Could you check a few things on this drawing? It's one solid part, dimensions in mm from its lowest x, y, z. Coordinates: 2 decimals unless noted, no trailing zeros. Order: outer loops, then holes, each group sorted by start corner. A loop starts at its lowest first (then second) coordinate and runs counter-clockwise, first axis right, second up. Notation, with made-up numbers: (71.5, 62.25) -> (127.5, 62.25) arc R20 cw to (127.5, 93.25) -> close; hole circle Ø9 at (77, -25). An arc over 180 degrees is marked (long way). Answer as CSV lines item,"result".
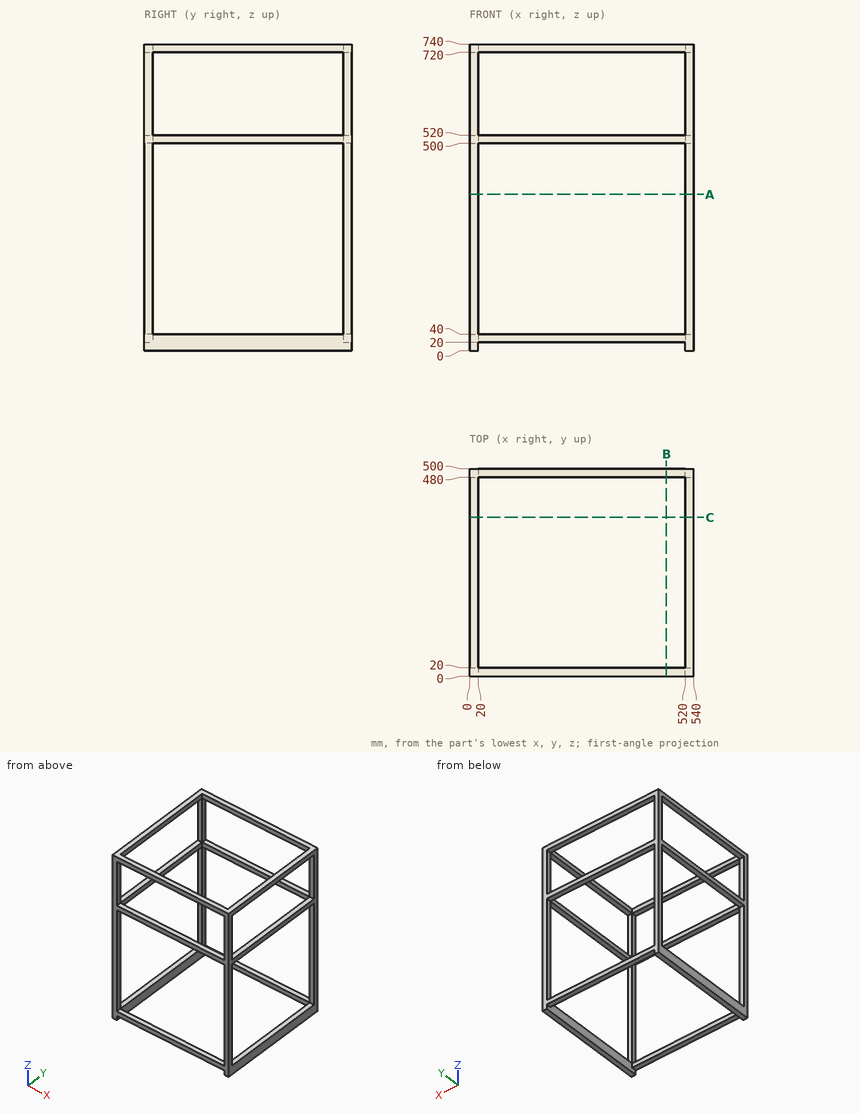
Q1. For P1, Ø22, axis at x = 177, y = 492, coming from the -Z side, with a flat end and sliding along its axis, tell me the tip position at first contact or that it passes through.
Solution:
P1,"z = 20"
Q2. Imagine slicing it at B-B (x = 474.5). List the corners of the cut face in (y, z) for me, and give its area (3 significant figures).
Solution:
outline,"(0, 20) -> (20, 20) -> (20, 40) -> (0, 40) -> close; (0, 500) -> (20, 500) -> (20, 520) -> (0, 520) -> close; (0, 720) -> (20, 720) -> (20, 740) -> (0, 740) -> close; (480, 20) -> (500, 20) -> (500, 40) -> (480, 40) -> close; (480, 500) -> (500, 500) -> (500, 520) -> (480, 520) -> close; (480, 720) -> (500, 720) -> (500, 740) -> (480, 740) -> close"
area,"2,400 mm2"
Q3. Imagine slicing it at A-A (z = 377.5). List the corners of the cut face in (x, y) for me.
Solution:
outline,"(0, 0) -> (20, 0) -> (20, 20) -> (0, 20) -> close; (0, 480) -> (20, 480) -> (20, 500) -> (0, 500) -> close; (520, 0) -> (540, 0) -> (540, 20) -> (520, 20) -> close; (520, 480) -> (540, 480) -> (540, 500) -> (520, 500) -> close"
Q4. If I drill on line 1 (Y direction, x = 24, z = 513.5), over which ranges is the centre line in solid material (lowest first)?
Solution:
line 1,"0 to 20, 480 to 500"
Q5. Imagine slicing it at C-C (y = 382.5). List the corners of the cut face in (x, z) for me.
Solution:
outline,"(0, 0) -> (20, 0) -> (20, 40) -> (0, 40) -> close; (0, 500) -> (20, 500) -> (20, 520) -> (0, 520) -> close; (0, 720) -> (20, 720) -> (20, 740) -> (0, 740) -> close; (520, 0) -> (540, 0) -> (540, 40) -> (520, 40) -> close; (520, 500) -> (540, 500) -> (540, 520) -> (520, 520) -> close; (520, 720) -> (540, 720) -> (540, 740) -> (520, 740) -> close"
